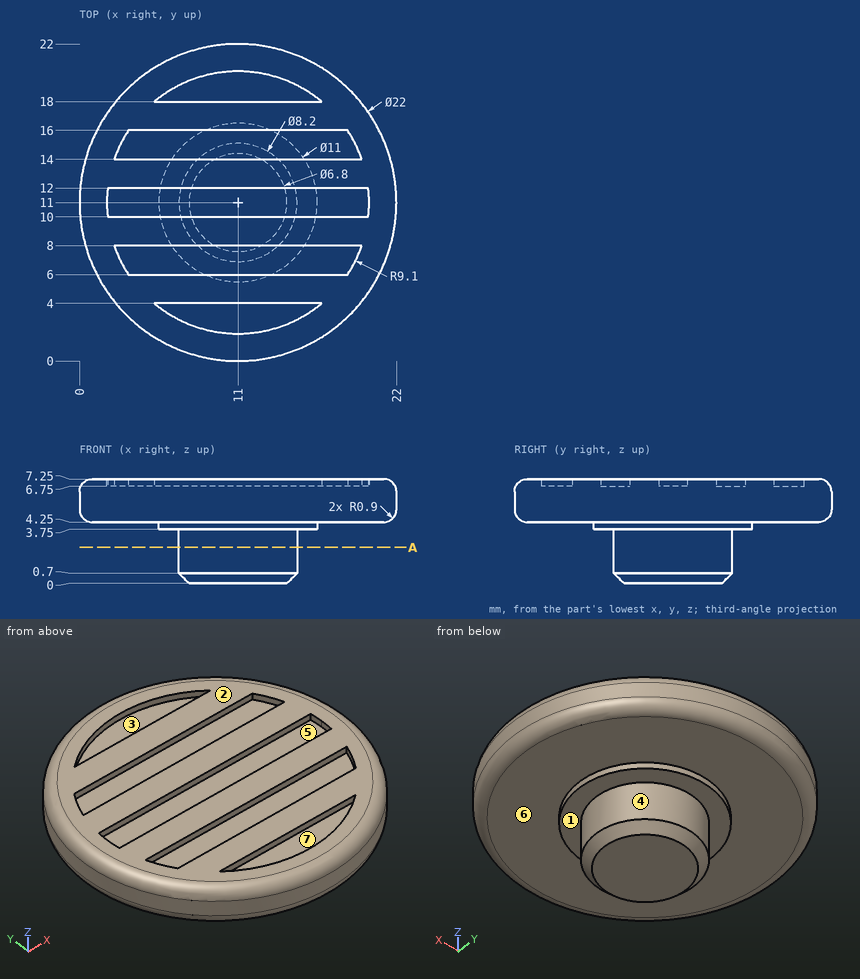
Verification items for this drawing (mm, ordinates from the low corner). A direction names the side the tool comes from. Coordinates: 2 decimals unless noted, no trailing zeros. Order: outer loops, then holes, each group sorted by start corner. A loop starts at its lowest first (then second) coordinate and runs counter-clockwise, first axis right, second up. Notation, with made-up numbers: M 21.25,89.5 L 39.25,89.5 A19 ccw 39.25,96.5 Z; hole C -13.5,-9.75 d5. An arc over 180 degrees is marked long. Answer as a JSON object with one key per item and string values.
Q1. Release check for a two-part mould opening along Y. For the marked faces 4, 5, 6 and 7 record: released by +Y, released by -Y, zero draft, split by the parting line, or undercut.
Results are:
{"face 4": "split by the parting line", "face 5": "undercut", "face 6": "zero draft", "face 7": "undercut"}
Q2. Depth check by flat-ended pin: pin 1 Ø0.6 at (x, z) = (9, 7) entering from -Y; pin 2 Ø10 at (x, y) = (19, 14) entering from -Z; pin 3 Ø1 at (y, z) = (14.5, 3.5) entering from -X. Enter the tip coordinate at first touch or a pass-through.
Results are:
{"pin 1": "stops at y = 0.24", "pin 2": "stops at z = 0.14", "pin 3": "stops at x = 6.43"}
Q3. Tool access check on the marked faces 1, 2 and 3. Record the directions out of +Z, -Z, +X, -X, +Y, -Y that give a thin tool (end or side, any length) a straight path to the whole face; none if there is none.
Results are:
{"face 1": "-Z", "face 2": "+Z, +X, -X, +Y, -Y", "face 3": "+Z"}
Q4. Cross-section at A-A on z = 2.5. Record the cut outline in (x, y), and give its area (3 significant figures).
Results are:
{"outline": "C 11,11 d8.2", "area": "52.8 mm²"}
Q5. Scan lines: line 1 (Z direction, x = 15.25, y = 15.75); line 2 (Z direction, x = 6.5, y = 4.75); line 3 (Y direction, x = 3, z = 5.25). Record each from-to range of solid material in increasing order.
Results are:
{"line 1": "z = 4.25 to 6.75", "line 2": "z = 4.25 to 7.25", "line 3": "y = 3.45 to 18.55"}
